Job drawing, mm, ordinate dimensions from the low corner. One solid piece. Give positions to 0.01 mm unless a question says otherwise; leave off trailing zeros. Write each loop counter-clockwise with the first axis right and the second up, starting at its lowest first coordinate (ties: lowest second). Pieces come first, ordered by that corner, then holes. Notation, with made-up numbers: (-30.5, 49.5) - (-17.5, 49.5) arc R25 cw to (-17.5, 68.5) - close; hole circle Ø11 at (3.25, -4.5). An arc over 180 degrees is marked (long way). Use a Markdown table: item, result. Add a question column.
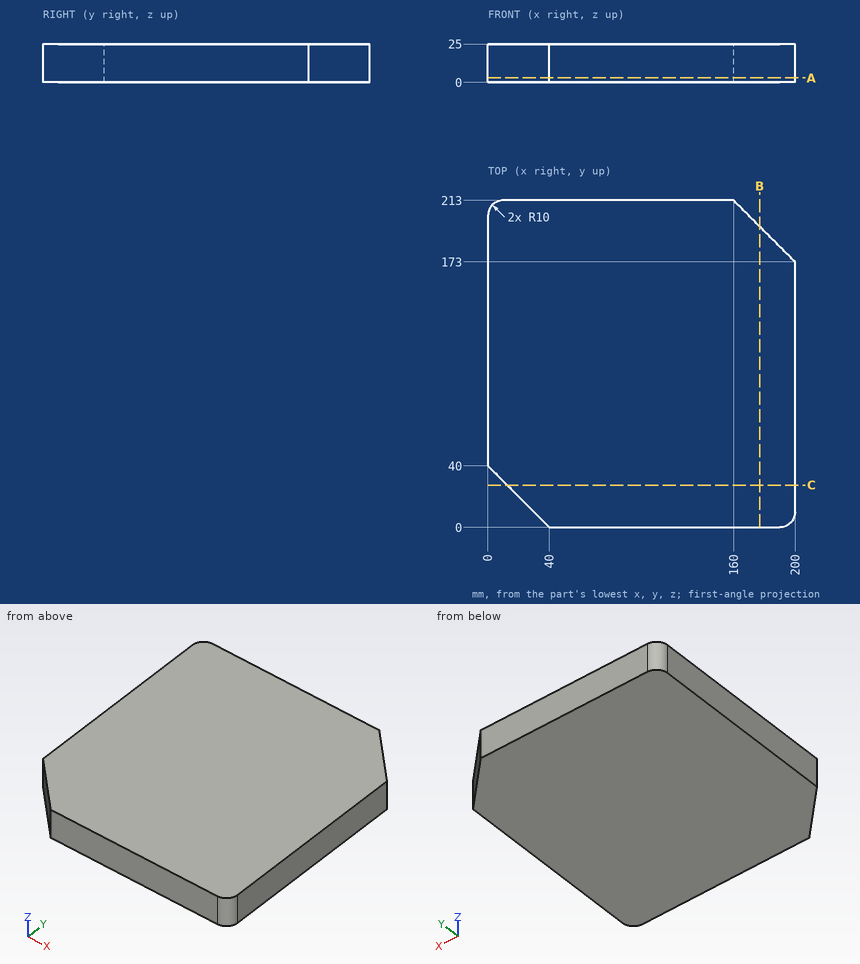
(1) Probe probe 1 along X at (y, z) = (11, 7.75); probe 2 along Y at (x, z) = (188, 17.5); probe 3 along X at (y, z) = (202, 8). List the from-to ranges inside material, lowest first. Write a range as [from, to].
(2) Band-saw the part on B-B (x = 177). Write the cut outline in (y, z).
(3) Band-saw the part on A-A (z = 3). Write the cut outline in (x, y), then the cut area to 3 significant figures.
(4) Flat gauge pin, fed straight in: pin 1 (3 mm diameter, centred on x = 22.5, z = 13.5, fed in from -Y). Where does the tip first touch, or does it go through?
(5) Band-saw the part on C-C (y = 27.5). Write the cut outline in (x, z).
Model answer:
| question | item | result |
|---|---|---|
| 1 | probe 1 | x = [29, 200] |
| 1 | probe 2 | y = [0, 185] |
| 1 | probe 3 | x = [0, 171] |
| 2 | outline | (0, 0) - (196, 0) - (196, 25) - (0, 25) - close |
| 3 | outline | (0, 40) - (40, 0) - (190, 0) arc R10 ccw to (200, 10) - (200, 173) - (160, 213) - (10, 213) arc R10 ccw to (0, 203) - close |
| 3 | area | 41,000 mm^2 |
| 4 | pin 1 | stops at y = 16 |
| 5 | outline | (12.5, 0) - (200, 0) - (200, 25) - (12.5, 25) - close |
